Source: CAD feature listing. Evaluate the final solid. Frame: model axes, mm. A direction names the side the tool comes from. Round coordinates to 2 decimals unless told otherwise and drop trailing zeros. Write each loop counter-clockwise with the first axis right and the second up, starting at its lowest first coordinate (ties: lowest second). Pieces come first, ordered by that corner, then holes. Notation, with made-up numbers: M 3,62.5 L 41,62.5 A26 cw 41,93.5 Z; hole C -21,32 d7. An arc over 180 degrees is marked long. Use a Markdown table: item, result.
```python
from build123d import *

# Parameters (mm, degrees)
BOSS_EXTRUDE1_DEPTH = 38.1
SHELL2_T            = -3.175
SKETCH2_W           = 279.4
SKETCH2_H           = 279.4
CUT_EXTRUDE1_DEPTH  = 73.025


with BuildPart() as part:
    # Sketch1 → Boss-Extrude1 (new body, symmetric)
    with BuildSketch(Plane.XY):
        Polygon((-152.4, 146.05), (-152.4, -146.05), (152.4, -146.05), (152.4, 146.05), (355.6, 336.55), (-355.6, 336.55), align=None)
    extrude(amount=BOSS_EXTRUDE1_DEPTH, both=True)

    # Shell2
    shell2_openings = [part.faces().sort_by_distance(p)[0] for p in [
        (0, 336.55, 0),
    ]]
    offset(amount=SHELL2_T, openings=shell2_openings, kind=Kind.INTERSECTION)

    # Sketch2 → Cut-Extrude1 (cut)
    with BuildSketch(Plane.XY.offset(38.1)):
        with Locations((0, 6.35)):
            Rectangle(SKETCH2_W, SKETCH2_H)
        Polygon((-350.957787584, 336.55), (-323.864454251, 311.15), (323.864454251, 311.15), (350.957787584, 336.55), align=None)
    extrude(amount=-CUT_EXTRUDE1_DEPTH, mode=Mode.SUBTRACT)


solid = part.part
```
Q1. Reachability of faces 1 (the flat face through (152.4, -2, 1)), 2 (the flat face through (-152.4, 2, 1)), 3 (the flat face through (-5, 152, -38.1)), 4 (the flat face through (149.225, 0, 0)) from +Z, -Z, +X, -X, +Y, -Y: full face, straight path, thin tool, end or side. Return the list, or none.
Results are:
| item | result |
|---|---|
| face 1 | +Z, -Z, +X, -Y |
| face 2 | +Z, -Z, -X, -Y |
| face 3 | -Z, +X, -X, +Y, -Y |
| face 4 | +Y |
Q2. First-contact query: pin 1 Ø3 at (y, z) = (188, -15.5) entering from +X; pin 2 Ø3.5 at (y, z) = (-57.5, 37) entering from -X; pin 3 Ø6 at (x, z) = (259, 5) entering from -Y (3 decimals). Flat tips, straight axial feed; report the tip coordinate or a pass-through.
Results are:
| item | result |
|---|---|
| pin 1 | x = 198.75 |
| pin 2 | x = -152.4 |
| pin 3 | y = 243.175 |
Q3. Line query: L1, parallel to X at y = -54.5, z = -14.5 (3 decimals); L2, parallel to Z at x = -198, y = 264.5 (3 decimals); L3, parallel to Y at x = 149, z = 29 (3 decimals). Output: solid intervals per line, ascending.
Results are:
| item | result |
|---|---|
| L1 | -152.4 to -149.225, 149.225 to 152.4 |
| L2 | -38.1 to -34.925, 34.925 to 38.1 |
| L3 | -146.05 to -142.875 |
Q4. Section D-D on y = 294.5. Return loops of the section in (x, z) (3 decimals), plus the area to 4 significant figures.
Results are:
| item | result |
|---|---|
| outline | M -310.747,-38.1 L 310.747,-38.1 L 310.747,38.1 L -310.747,38.1 Z; hole M -306.104,-34.925 L 306.104,-34.925 L 306.104,34.925 L -306.104,34.925 Z |
| area | 4,595 mm^2 |
Q5. Section B-B on z = 10. Return loops of the section in (x, y) (3 decimals).
Results are:
| item | result |
|---|---|
| outline | M -355.6,336.55 L -152.4,146.05 L -152.4,-146.05 L 152.4,-146.05 L 152.4,146.05 L 355.6,336.55 L 350.958,336.55 L 149.225,147.426 L 149.225,-142.875 L -149.225,-142.875 L -149.225,147.426 L -350.958,336.55 Z |
Q6. Section A-A on x = 30.5. Return loops of the section in (y, z) (3 decimals).
Results are:
| item | result |
|---|---|
| outline | M -146.05,-38.1 L 336.55,-38.1 L 336.55,-34.925 L -142.875,-34.925 L -142.875,34.925 L -133.35,34.925 L -133.35,38.1 L -146.05,38.1 Z; M 146.05,34.925 L 311.15,34.925 L 311.15,38.1 L 146.05,38.1 Z |
Q7. Section C-C on y = -93. Return loops of the section in (x, z) (3 decimals), plus the area to 3 significant figures.
Results are:
| item | result |
|---|---|
| outline | M -152.4,-38.1 L 152.4,-38.1 L 152.4,38.1 L 139.7,38.1 L 139.7,34.925 L 149.225,34.925 L 149.225,-34.925 L -149.225,-34.925 L -149.225,34.925 L -139.7,34.925 L -139.7,38.1 L -152.4,38.1 Z |
| area | 1,490 mm^2 |
